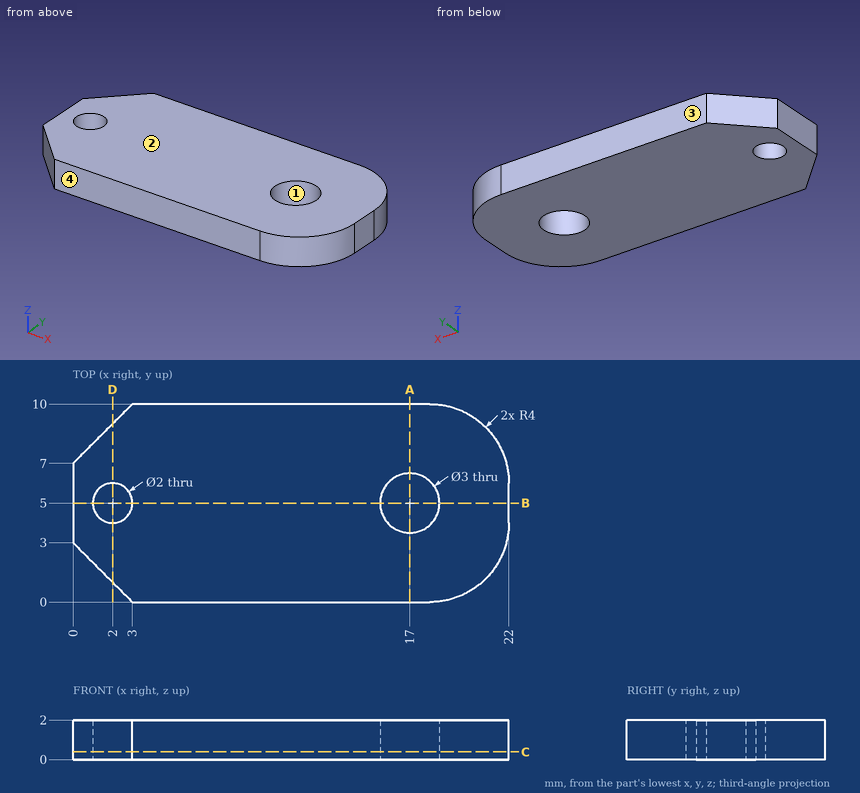
Part print with two shaded views. Sizes in mm from the minimum x, y, z corner. Coordinates: 2 decimals unless noted, no trailing zeros. Order: outer loops, then holes, each group sorted by start corner. A loop starts at its lowest first (then second) coordinate and runs counter-clockwise, first axis right, second up. Notation, with made-up numbers: (20.5, 29.5) - (43.5, 29.5) arc R35 cw to (43.5, 68.5) - close; hole circle Ø3 at (13.25, -2). An arc over 180 degrees is marked (long way). Answer in a Markdown table with one row per item.
1. Drill centre lines: L1, parallel to X at y = 5.75, z = 1.5; L2, parallel to X at y = 4.5, z = 0.35; L3, parallel to Y at x = 17, z = 0.7. Where is each one in solid material? Low to high. Write a range as from..to.
Answer:
| item | result |
|---|---|
| L1 | 0..1.34, 2.66..15.7, 18.3..22 |
| L2 | 0..1.13, 2.87..15.59, 18.41..22 |
| L3 | 0..3.5, 6.5..10 |
2. Slice it at A-A, the plane x = 17. List the corners of the cut face in (y, z).
Answer:
| item | result |
|---|---|
| outline | (0, 0) - (3.5, 0) - (3.5, 2) - (0, 2) - close; (6.5, 0) - (10, 0) - (10, 2) - (6.5, 2) - close |
3. Slice it at C-C, the plane z = 0.4. List the corners of the cut face in (x, y).
Answer:
| item | result |
|---|---|
| outline | (0, 3) - (3, 0) - (18, 0) arc R4 ccw to (22, 4) - (22, 6) arc R4 ccw to (18, 10) - (3, 10) - (0, 7) - close; hole circle Ø2 at (2, 5); hole circle Ø3 at (17, 5) |
4. Slice it at D-D, the plane x = 2. List the corners of the cut face in (y, z), then the cut area to 3 significant figures.
Answer:
| item | result |
|---|---|
| outline | (1, 0) - (4, 0) - (4, 2) - (1, 2) - close; (6, 0) - (9, 0) - (9, 2) - (6, 2) - close |
| area | 12.0 mm² |
5. Flat gauge pin, fed straight in: P1, Ø3, axis at x = 2, y = 5, coming from the -Z side. Where does the tip first touch, or does it go through?
Answer:
| item | result |
|---|---|
| P1 | z = 0 |
6. Slice it at B-B, the plane y = 5. List the corners of the cut face in (x, z).
Answer:
| item | result |
|---|---|
| outline | (0, 0) - (1, 0) - (1, 2) - (0, 2) - close; (3, 0) - (15.5, 0) - (15.5, 2) - (3, 2) - close; (18.5, 0) - (22, 0) - (22, 2) - (18.5, 2) - close |
7. Pull direction Y, two halves, no side cores. Call the marked faces 1, 2, 3 and 4: +Y half, -Y half, draft (parallel to the pull), parting line (faces both ways), or undercut.
Answer:
| item | result |
|---|---|
| face 1 | undercut |
| face 2 | draft |
| face 3 | +Y half |
| face 4 | -Y half |
